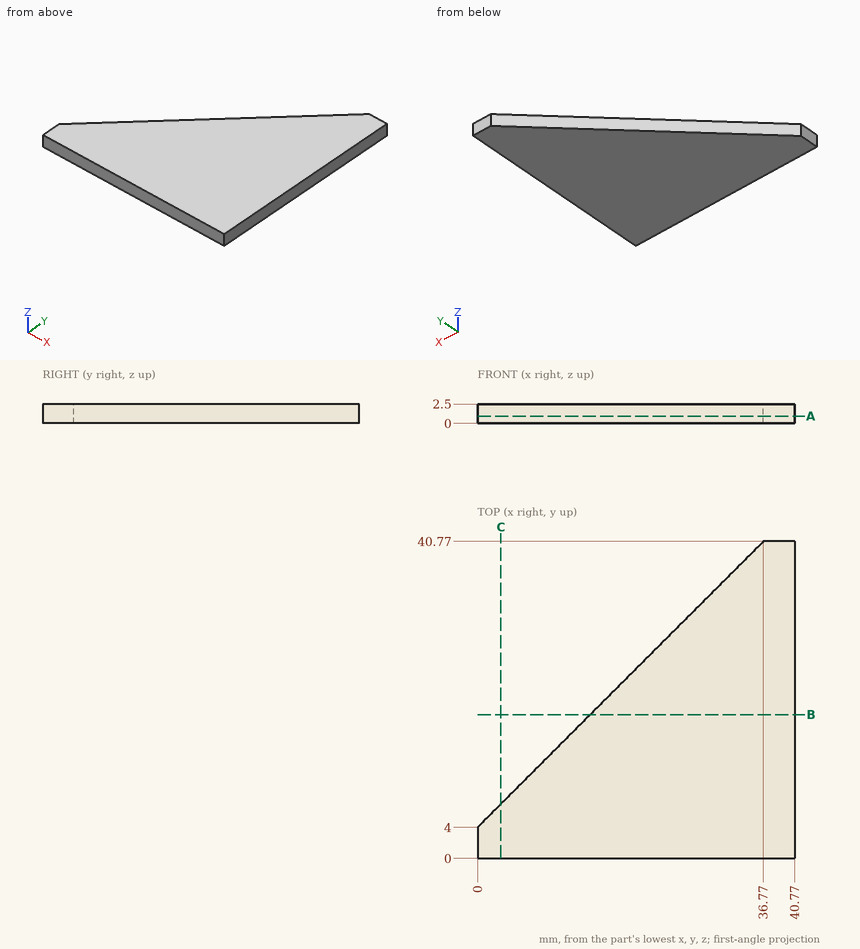
Here's the drawing with two shaded views (mm, measured from the low corner). I have some questions. Give positions to 0.01 mm unless a question says otherwise; leave off trailing zeros. Order: outer loops, then holes, each group sorted by start corner. A loop starts at its lowest first (then second) coordinate and runs counter-clockwise, first axis right, second up. Notation, with made-up numbers: (67.25, 60) - (98.25, 60) arc R32 ccw to (98.25, 87) - close; hole circle Ø4 at (28, 29). An arc over 180 degrees is marked (long way). Use a Markdown table: item, result. Add a question column.
Q1. If we section it at A-A on z = 0.95: Write out the boundary of the cut face in (x, y).
Q2. I'm going to push a flat-ended pin straight in: pin 1 (1 mm diameter, centred on y = 35, z = 2, fed in from -X). Where does the tip first touch, or does it pass through?
Q3. If we section it at B-B on y = 18.5: Write out the boundary of the cut face in (x, z).
Q4. Please list where these lines run through material, in increasing order: line 1 along Y through (x, z) = (34, 2.2); line 2 along Y through (x, z) = (25, 1.85); line 3 along X through (y, z) = (24, 1.35).
Q5. If we section it at C-C on x = 3: Write out the boundary of the cut face in (y, z).
Answers follow:
| question | item | result |
|---|---|---|
| 1 | outline | (0, 0) - (40.77, 0) - (40.77, 40.77) - (36.77, 40.77) - (0, 4) - close |
| 2 | pin 1 | stops at x = 30.5 |
| 3 | outline | (14.5, 0) - (40.77, 0) - (40.77, 2.5) - (14.5, 2.5) - close |
| 4 | line 1 | y = 0 to 38 |
| 4 | line 2 | y = 0 to 29 |
| 4 | line 3 | x = 20 to 40.77 |
| 5 | outline | (0, 0) - (7, 0) - (7, 2.5) - (0, 2.5) - close |
